The model under review builds one solid part; all positions refer to its coordinate system, in mm. Face numbers are marked on the shaded views. A direction names the side the tool comes from. Round coordinates to 2 decimals unless told otherwise and drop trailing zeros. Loops run counter-clockwise (first coordinate to the right, second up) from the corner with the lowest first, then second, coordinate; pieces in that order, holes last. Notation, with made-up numbers: M 51,2.5 L 62,2.5 A15 cw 62,12.5 Z; hole C -25.5,65 d8. An arc over 180 degrees is marked long. Answer as a JSON object with one key per item and string values. Group by question number.
Item 1: Consider section C-C (z = -3.5). Give the boundary of the cut face in (x, y), and give its area (3 significant figures).
Item 2: To check wall thickness, follow line 1 (Z direction, x = 0, y = -9.25); line 2 (Z direction, x = -6, y = -13.5); line 3 (X direction, y = -19.5, z = 115.5). State the ranges of each line that lie inside material, in increasing order.
Item 3: Consider section D-D (z = 118). Give the boundary of the cut face in (x, y).
Item 4: Consider section A-A (x = 0). Give the boundary of the cut face in (y, z), and give its area (3 significant figures).
Item 5: The part is to be moulded in two halves that separate along Z. For the marked faces 1 and 2, say which applies: +Z half, -Z half, draft (parallel to the pull), parting line (faces both ways), or undercut.
Item 6: Tool access review of the marked faces 3 and 4: name each direction out of +Z, -Z, +X, -X, +Y, -Y from which nothing blocks a thin tool from reaching the whole face with its end or side.
Item 7: Insertion check: P1, Ø5, axis at y = -4, z = 12, coming from the +X side; P2, Ø4, axis at x = 24, y = -12, coming from the -Z side; P3, Ø1.5, axis at x = 8, y = -9.5, coming from the +Z side. Each pin has a flat end and moves straight along its axis. Give the tip position at first contact, or say it passes through.
Item 8: Consider section B-B (y = -3.5). Give the boundary of the cut face in (x, z).
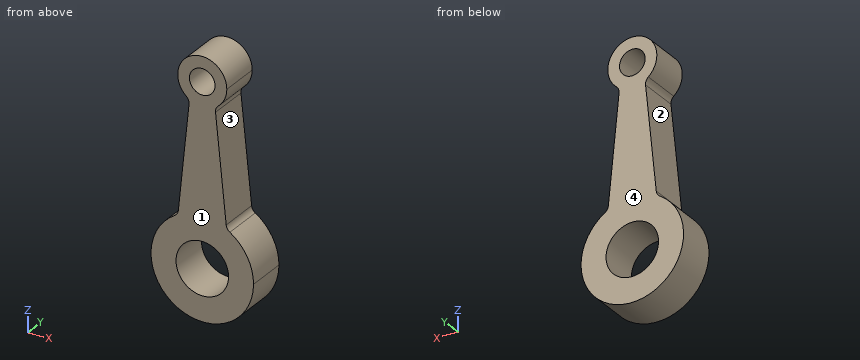
```python
from build123d import *

# Parameters (mm, degrees)
F0_R     = 16.628387
F0_R_2   = 8.110112
F1_DEPTH = 25.4
F2_R     = 5.08


with BuildPart() as f1:
    # F0 (on Front) → F1 (new body)
    with BuildSketch(Plane.XZ):
        with BuildLine():
            ThreePointArc((-15.411044, 28.557638), (-16.627416, -27.866969), (32.450562, 0))
            ThreePointArc((32.450562, 0), (27.866969, 16.627416), (15.411044, 28.557638))
            ThreePointArc((15.411044, 28.557638), (0, 32.450562), (-15.411044, 28.557638))
        make_face()
        Circle(F0_R, mode=Mode.SUBTRACT)
        with BuildLine():
            ThreePointArc((-15.411044, 28.557638), (0, 32.450562), (15.411044, 28.557638))
            Line((15.411044, 28.557638), (8.096426, 100.779159))
            ThreePointArc((8.096426, 100.779159), (0, 98.503095), (-8.096426, 100.779159))
            Line((-8.096426, 100.779159), (-15.411044, 28.557638))
        make_face()
        with BuildLine():
            ThreePointArc((-8.096426, 100.779159), (0, 98.503095), (8.096426, 100.779159))
            ThreePointArc((8.096426, 100.779159), (13.550753, 106.437659), (15.53836, 114.041455))
            ThreePointArc((15.53836, 114.041455), (-7.603796, 127.592208), (-8.096426, 100.779159))
        make_face()
        with Locations((0, 114.041455)):
            Circle(F0_R_2, mode=Mode.SUBTRACT)
    extrude(amount=F1_DEPTH)

    # F2
    f2_edges = [f1.edges().sort_by_distance(p)[0] for p in [
        (15.411044, -12.7, 28.557638),
        (-15.411044, -12.7, 28.557638),
        (-8.096426, -12.7, 100.779159),
        (8.096426, -12.7, 100.779159),
    ]]
    fillet(f2_edges, radius=F2_R)


solid = f1.part
```
Geometry results:
{
 "1": {"outline": "M -32.26,-25.4 L -16.26,-25.4 L -16.26,0 L -32.26,0 Z; M 16.26,-25.4 L 32.26,-25.4 L 32.26,0 L 16.26,0 Z", "area": "813 mm^2"},
 "2": {"line 1": "z = -32.45 to -16.63, 16.63 to 105.93, 122.15 to 129.58", "line 2": "z = -31.89 to -15.51, 15.51 to 108.58, 119.5 to 128.37", "line 3": "x = -15.47 to -7.98, 7.98 to 15.47"},
 "3": {"outline": "M -15.03,-25.4 L -7.08,-25.4 L -7.08,0 L -15.03,0 Z; M 7.08,-25.4 L 15.03,-25.4 L 15.03,0 L 7.08,0 Z"},
 "4": {"outline": "M -25.4,-32.45 L 0,-32.45 L 0,-16.63 L -25.4,-16.63 Z; M -25.4,16.63 L 0,16.63 L 0,105.93 L -25.4,105.93 Z; M -25.4,122.15 L 0,122.15 L 0,129.58 L -25.4,129.58 Z", "area": "2,860 mm^2"},
 "5": {"face 1": "draft", "face 2": "undercut"},
 "6": {"face 3": "+X, +Y, -Y", "face 4": "+Z, -Z, +X, -X, +Y"},
 "7": {"P1": "stops at x = 31.03", "P2": "stops at z = -23.85", "P3": "stops at z = 127.78"},
 "8": {"outline": "M -17.47,27.35 A32.45 ccw long 32.45,0 A32.45 ccw 17.47,27.35 A5.08 cw 15.15,31.11 L 8.39,97.9 A5.08 cw 10.13,102.26 A15.54 ccw long -10.13,102.26 A5.08 cw -8.39,97.9 L -15.15,31.11 A5.08 cw Z; hole C 0,0 d33.26; hole C 0,114.04 d16.22"}
}
